Verification items for the finished model (mm, model axes). A direction names the side the tool comes from. Round coordinates to 2 decimals unless told otherwise and drop trailing zeros. Loops run counter-clockwise (first coordinate to the right, second up) from the corner with the lowest first, then second, coordinate; pieces in that order, holes last. Notation, with made-up numbers: (3.5, 48.25) -> (32.5, 48.25) arc R20 cw to (32.5, 83.25) -> close; hole circle Ø4 at (-19, 29). An arc over 180 degrees is marked (long way). Use a Markdown table: item, result. Add a question column.
```python
from build123d import *

# Parameters (mm, degrees)
SKETCH2_W          = 32.050318883
SKETCH2_H          = 65.476021051
SKETCH2_W_2        = 24.596756352
SKETCH2_H_2        = 67.490667853
CUT_EXTRUDE1_DEPTH = 100
CUT_EXTRUDE2_REACH = 1868.397
SKETCH3_R          = 12.5


with BuildPart() as part:
    # Sketch1 → Revolve1 (revolve)
    with BuildSketch(Plane(origin=(0, 0, 0), x_dir=(0, 0, -1), z_dir=(1, 0, 0)), mode=Mode.PRIVATE) as revolve1_sk:
        Polygon((0, 0), (1837.5, 0), (1837.5, -25), (450, -25), (450, -225), (325, -225), (325, -100), (125, -100), (125, -225), (0, -225), align=None)
    revolve(revolve1_sk.sketch.rotate(Axis((0, 0, 0), (0, 0, -1)), 270), axis=Axis((0, 0, 0), (0, 0, -1)))

    # Sketch2 → Cut-Extrude1 (cut)
    with BuildSketch(Plane(origin=(0, 0, -1837.5), x_dir=(-1, 0, 0), z_dir=(0, 0, -1))):
        with Locations((-28.525159442, 1.561413984)):
            Rectangle(SKETCH2_W, SKETCH2_H)
        with Locations((24.798378176, 2.232962919)):
            Rectangle(SKETCH2_W_2, SKETCH2_H_2)
    extrude(amount=-CUT_EXTRUDE1_DEPTH, mode=Mode.SUBTRACT)

    # Sketch3 → Cut-Extrude2 (cut, up to next)
    with BuildSketch(Plane(origin=(12.5, 0, 0), x_dir=(0, 0, -1), z_dir=(1, 0, 0)), mode=Mode.PRIVATE) as cut_extrude2_sk1:
        with Locations((1787.5, 0)):
            Circle(SKETCH3_R)
    cut_extrude2_tool1 = extrude(cut_extrude2_sk1.sketch, amount=-CUT_EXTRUDE2_REACH, mode=Mode.PRIVATE) & part.part
    add(cut_extrude2_tool1.solids().sort_by_distance((12.5, 0, -1787.5))[0], mode=Mode.SUBTRACT)


solid = part.part
```
1) Release check for a two-part mould opening along Z. For faces 1 (the face through (3, 47, -450)), 2 (the face through (-224.782, -9.893, -386.625)), 3 (the face through (95.38, -30.04, -223.6)), 4 (the face through (-97, 47, -125)) record: released by +Z, released by -Z, zero draft, split by the parting line, or undercut.
2) Thickness scan on line 1 (Z direction, x = 134, y = 140.5); line 2 (Y direction, x = -0.25, z = -1787.5); line 3 (Z direction, x = -56, y = 19). Record the ranges inside material, lowest first.
3) Sectioned sample at D-D on z = -830.5. Enter the section's corners in (x, y), then the cut area to 3 significant figures.
4) Access from +Z, -Z, +X, -X, +Y, -Y to the whole of each face (thin tool, end or side, straight path). Record for faces 5 (the face through (-3, -3, 0)), 6 (the face through (97, 47, -325)), 7 (the face through (12.5, -5.1, -1799.3)), 8 (the face through (-12.5, -5.1, -1799.3)), 9 (the face through (-5.42, 24.406, -1134.038)).
5) Sectioned sample at A-A on y = -143. Enter the section's corners in (x, z).
6) Sectioned sample at C-C on x = -72. Enter the section's corners in (y, z).
7) Sectioned sample at B-B on x = 169.5. Enter the section's corners in (y, z), then the cut area to 3 significant figures.
8) Go/stop test with flat-tipped pins: pin 1 (4 mm diameter, centred on x = -7, z = -1362.5, fed in from -Y); pin 2 (3 mm diameter, centred on y = -27.5, z = -1428.5, fed in from -X); pin 3 (4 mm diameter, centred on x = -172.5, z = -441.5, fed in from -Y); pin 4 (13 mm diameter, centred on y = -6, z = -1811, fed in from -X). Record where each tip stops, or that it passes through.
Geometry results:
| question | item | result |
|---|---|---|
| 1 | face 1 | released by -Z |
| 1 | face 2 | zero draft |
| 1 | face 3 | undercut |
| 1 | face 4 | undercut |
| 2 | line 1 | -450 to -325, -125 to 0 |
| 2 | line 2 | -25 to -12.5, 12.5 to 25 |
| 2 | line 3 | -450 to 0 |
| 3 | outline | circle Ø50 at (0, 0) |
| 3 | area | 1,960 mm^2 |
| 4 | face 5 | +Z, +X, -X, +Y, -Y |
| 4 | face 6 | none |
| 4 | face 7 | -Z, +X, +Y, -Y |
| 4 | face 8 | -Z, -X, +Y, -Y |
| 4 | face 9 | -Z |
| 5 | outline | (-173.71, -450) -> (173.71, -450) -> (173.71, -325) -> (-173.71, -325) -> close; (-173.71, -125) -> (173.71, -125) -> (173.71, 0) -> (-173.71, 0) -> close |
| 6 | outline | (-213.17, -450) -> (213.17, -450) -> (213.17, -325) -> (69.4, -325) -> (69.4, -125) -> (213.17, -125) -> (213.17, 0) -> (-213.17, 0) -> (-213.17, -125) -> (-69.4, -125) -> (-69.4, -325) -> (-213.17, -325) -> close |
| 7 | outline | (-147.97, -450) -> (147.97, -450) -> (147.97, -325) -> (-147.97, -325) -> close; (-147.97, -125) -> (147.97, -125) -> (147.97, 0) -> (-147.97, 0) -> close |
| 7 | area | 74,000 mm^2 |
| 8 | pin 1 | y = -24.49 |
| 8 | pin 2 | through |
| 8 | pin 3 | y = -146.82 |
| 8 | pin 4 | x = -12.5 |
